Read the model definition and answer for the solid it produces. Units are mm, in the model's axes. A direction names the side the tool comes from. Coordinates: 2 decimals unless noted, no trailing zeros. Write each loop counter-clockwise with the first axis right and the second up, starting at its lowest first coordinate (ties: lowest second). Pieces come first, ordered by that corner, then holes. Notation, with made-up numbers: (0.5, 11.25) - (7.5, 11.25) arc R28 ccw to (7.5, 30.25) - close; hole circle Ø2 at (17, 42). An arc over 180 degrees is marked (long way). Use a Markdown table: item, result.
from build123d import *

# Parameters (mm, degrees)
F1_DEPTH = 6.35


with BuildPart() as f1:
    # F0 (on Top) → F1 (new body)
    with BuildSketch(Plane.XY):
        Polygon((-2.899504, 0.53663), (-2.899504, 0), (3.129742, 0), (3.129742, 0.5334), (5.253811, 0.5334), (5.253811, 3.175), (-5.253811, 3.175), (-5.253811, 0.53663), align=None)
        Polygon((3.129742, 0), (-2.899504, 0), (-2.899504, -0.53663), (-5.253811, -0.53663), (-5.253811, -3.175), (5.253811, -3.175), (5.253811, -0.5334), (3.129742, -0.5334), align=None)
        Polygon((5.253811, -0.5334), (5.253811, -3.175), (5.253811, -3.81), (6.396811, -3.81), (7.240531, -0.5334), align=None)
        Polygon((5.253811, 3.81), (5.253811, 3.175), (5.253811, 0.5334), (7.240531, 0.5334), (6.396811, 3.81), align=None)
        Polygon((-6.396811, 3.81), (-7.437509, 0.53663), (-5.253811, 0.53663), (-5.253811, 3.175), (-5.253811, 3.81), align=None)
        Polygon((-5.253811, -0.53663), (-7.437509, -0.53663), (-6.396811, -3.81), (-5.253811, -3.81), (-5.253811, -3.175), align=None)
    extrude(amount=F1_DEPTH)


solid = f1.part
(1) For faces 5 (the flat face through (5, 0.533, 3)), 6 (the flat face through (-5, -0.537, 3)), 7 (the flat face through (6, -3.81, 3)), determine the directions among +Z, -Z, +X, -X, +Y, -Y from which every point of the face is accessible in a straight line to the end or side of a thin tool.
Report:
| item | result |
|---|---|
| face 5 | +Z, -Z, +X |
| face 6 | +Z, -Z, -X |
| face 7 | +Z, -Z, +X, -X, -Y |
(2) A cutting plane is placed at B-B, the plane z = 1. Write down the section's boundary in (x, y) (1 decimal).
Report:
| item | result |
|---|---|
| outline | (-7.4, -0.5) - (-6.4, -3.8) - (-5.3, -3.8) - (-5.3, -3.2) - (5.3, -3.2) - (5.3, -3.8) - (6.4, -3.8) - (7.2, -0.5) - (3.1, -0.5) - (3.1, 0.5) - (7.2, 0.5) - (6.4, 3.8) - (5.3, 3.8) - (5.3, 3.2) - (-5.3, 3.2) - (-5.3, 3.8) - (-6.4, 3.8) - (-7.4, 0.5) - (-2.9, 0.5) - (-2.9, -0.5) - close |
(3) Each of these flat-tipped pins is pushed along its axis until it touches: P1, Ø0.5, axis at y = 0, z = 4.5, coming from the +X side; P2, Ø3, axis at x = 2.5, z = 3.5, coming from the +Y side (3 decimals); P3, Ø3.5, axis at x = -4.5, z = 4.5, coming from the +Y side; P4, Ø2, axis at y = 2.5, z = 2, coming from the +X side. Where does it stop, or does it pass through?
Report:
| item | result |
|---|---|
| P1 | stops at x = 3.13 |
| P2 | stops at y = 3.175 |
| P3 | stops at y = 3.81 |
| P4 | stops at x = 6.99 |
(4) The mould has two halves that part along X. Classify faces 1 (the flat face through (-5, 0.537, 3)), 2 (the flat face through (0, -3.175, 3)), 3 (the flat face through (0, 3.175, 3)), 4 (the flat face through (-6.924, -2.15, 3.131)): pulls with the +X half, pulls with the -X half, needs draft (parallel to the pull), parting line crosses it, or undercut.
Report:
| item | result |
|---|---|
| face 1 | needs draft |
| face 2 | undercut |
| face 3 | undercut |
| face 4 | pulls with the -X half |
(5) A cutting plane is placed at D-D, the plane x = -0.5. Write down the section's boundary in (y, z) (3 decimals), and give its area (3 significant figures).
Report:
| item | result |
|---|---|
| outline | (-3.175, 0) - (3.175, 0) - (3.175, 6.35) - (-3.175, 6.35) - close |
| area | 40.3 mm² |
(6) Straight lines are drawn through the part: L1, parallel to Y at x = -3, z = 2.5 (3 decimals); L2, parallel to X at y = -0.25, z = 2; L3, parallel to Y at x = -1.5, z = 3 (3 decimals). For each, find the intervals that lie inside material, in ascending order.
Report:
| item | result |
|---|---|
| L1 | y = -3.175 to -0.537, 0.537 to 3.175 |
| L2 | x = -2.9 to 3.13 |
| L3 | y = -3.175 to 3.175 |
(7) A cutting plane is placed at C-C, the plane y = 1.25. Write down the section's boundary in (x, z), and give its area (3 significant figures).
Report:
| item | result |
|---|---|
| outline | (-7.21, 0) - (7.06, 0) - (7.06, 6.35) - (-7.21, 6.35) - close |
| area | 90.6 mm² |
(8) A cutting plane is placed at A-A, the plane x = -4.75. Write down the section's boundary in (y, z) (3 decimals), and give its area (3 significant figures).
Report:
| item | result |
|---|---|
| outline | (-3.175, 0) - (-0.537, 0) - (-0.537, 6.35) - (-3.175, 6.35) - close; (0.537, 0) - (3.175, 0) - (3.175, 6.35) - (0.537, 6.35) - close |
| area | 33.5 mm² |
